from build123d import *

# Parameters (mm, degrees)
F2_DEPTH = 9
F3_COUNT = 8
F4_ANGLE = -12.10395829
F5_R     = 1.5
F6_DEPTH = 9


with BuildPart() as f2:
    # F0 (on Top) → F2 (new body)
    with BuildSketch(Plane.XY):
        with BuildLine():
            ThreePointArc((3.6214284351, 1.6281359465), (-3.8823170623, -0.8325772028), (3.9705881895, 0))
            ThreePointArc((3.9705881895, 0), (3.8823170623, 0.8325772028), (3.6214284351, 1.6281359465))
        make_face()
        with BuildLine():
            ThreePointArc((3.6214284351, 1.6281359465), (3.8823170623, 0.8325772028), (3.9705881895, 0))
            Line((3.9705881895, 0), (4.974843229, 0))
            add(Edge.make_bspline(
                [(4.974843229, 0), (4.9801466314, 0.0001925881), (4.9946353816, 0.0007187334), (5.0515091084, 0.007901301), (5.1389720703, 0.0270949003), (5.2611962602, 0.0647089906), (5.4129160811, 0.1262103484), (5.5914935571, 0.2170132856), (5.7925834332, 0.3418264578), (6.0112959876, 0.5056653333), (6.2248108983, 0.6935311725), (6.3607565303, 0.8389400469), (6.4217785849, 0.9054272978)],
                knots=[0, 0, 0, 0, 0.0334564641, 0.0914021433, 0.1662094232, 0.2547225024, 0.3550868593, 0.4660438076, 0.5866667132, 0.7162364887, 0.8541740412, 0.9672633179, 0.9672633179, 0.9672633179, 0.9672633179], degree=3))
            ThreePointArc((6.4217785849, 0.9054272978), (6.3411178656, 1.3598760973), (6.2283392589, 1.8074370975))
            add(Edge.make_bspline(
                [(4.5373727694, 2.0399297793), (4.5422887796, 2.041928782), (4.5557191847, 2.0473900024), (4.6105368383, 2.0641600629), (4.698178928, 2.0825183873), (4.8250787688, 2.0983298636), (4.9886754487, 2.1044492916), (5.1887830997, 2.0948567755), (5.4233693532, 2.0634759551), (5.6900310606, 2.0037273789), (5.961804421, 1.9199333981), (6.1454202376, 1.843055654), (6.2283392589, 1.8074370975)],
                knots=[0, 0, 0, 0, 0.0334564641, 0.0914021433, 0.1662094232, 0.2547225024, 0.3550868593, 0.4660438076, 0.5866667132, 0.7162364887, 0.8541740412, 0.9672633179, 0.9672633179, 0.9672633179, 0.9672633179], degree=3))
            Line((4.5373727694, 2.0399297793), (3.6214284351, 1.6281359465))
        make_face()
    extrude(amount=F2_DEPTH)

    # F3: F2 ×8 about axis
    f3_axis = Axis((0, 0, 12.9622193053), (0, 0, 1))


with BuildPart() as f2_1:
    add(f2.part)
    for i in range(1, F3_COUNT):
        add(f2.part.rotate(f3_axis, i * 360 / F3_COUNT))


with BuildPart() as f2_2:
    # F4: moved
    add(f2_1.part.rotate(Axis((0, 0, 12.9622193053), (0, 0, 1)), F4_ANGLE))

    # F5 (on face) → F6 (cut, through all)
    with BuildSketch(Plane.XY.offset(9)):
        Circle(F5_R)
    extrude(amount=-F6_DEPTH, mode=Mode.SUBTRACT)


solid = f2_2.part
Could you check a few things on this model? Use its own coordinates, in mm. A direction names the side the tool comes from. Give positions to 0.01 mm unless a question says otherwise; leave off trailing zeros. Order: outer loops, then holes, each group sorted by start corner. A loop starts at its lowest first (then second) coordinate and runs counter-clockwise, first axis right, second up. Notation, with made-up numbers: (21, 38.25) - (52, 38.25) arc R31 ccw to (52, 70.25) - close; hole circle Ø4 at (-13, -34.75). An arc over 180 degrees is marked (long way). One line per question, with ' | ' between items. Start each with the question number.
Item 1: I want a section at C-C on y = -3.5. Give the number of separate pieces and of enclosed holes in the cut face, then the cut area to 3 significant figures.
Item 2: I want a section at A-A on y = 0. Write out the boundary of the cut face in (x, z).
Item 3: I'm going to push flat-ended pins straight in: pin 1 Ø1.5 at (x, z) = (-2.5, 6) entering from -Y; pin 2 Ø1.5 at (y, z) = (-2, 2.5) entering from -X; pin 3 Ø2 at (y, z) = (3, 7) entering from -X. Where does each tip first touch, or does it pass through?
Item 4: Thinking about a two-plate mould opening in Y: for faces 1 (the cylindrical face through (3.672, 1.51, 4.437)), 2 (the cylindrical face through (0.006, 6.485, 4.437)), 3 (the flat face through (-2.43, -3.76, 4.44)), which applies, pulls with the +Y half, pulls with the -Y half, needs draft (parallel to the pull), parting line crosses it, or undercut?
Item 5: For faces 4 (the cylindrical face through (-6.485, 0.006, 4.437)), 5 (the flat face through (-2.425, 3.75, 4.437)), 6 (the flat face through (3.76, -2.43, 4.44)), 7 (the flat face through (4.366, -0.936, 4.437)), 8 (the flat face through (2.425, -3.75, 4.437)), which set-ups out of +Z, -Z, +X, -X, +Y, -Y let a thin tool reach every point of the face, with its end or its side?
Item 6: I need wall thicknesses on probe 1 along Y at (x, z) = (0, 5.5); probe 2 along Y at (x, z) = (4.5, 3.25); probe 3 along X at (y, z) = (-0.5, 7.5). Which ranges of each line are inside material? Lowest first, please. Write a range as [from, to].
Verdict:
1) separate pieces: 3 | enclosed holes: 0 | area: 77.6 mm^2
2) outline: (-6.49, 0) - (-1.5, 0) - (-1.5, 9) - (-6.49, 9) - close; (1.5, 0) - (6.49, 0) - (6.49, 9) - (1.5, 9) - close
3) pin 1: y = -4.59 | pin 2: x = -4.24 | pin 3: x = -4.85
4) face 1: undercut | face 2: pulls with the +Y half | face 3: pulls with the -Y half
5) face 4: +Z, -Z, -X | face 5: +Z, -Z, +Y | face 6: +Z, -Z, +X | face 7: +Z, -Z | face 8: +Z, -Z, -Y
6) probe 1: [-6.49, -1.5], [1.5, 6.49] | probe 2: [-4.67, -3.09], [-0.97, 0.97], [3.09, 4.67] | probe 3: [-6.41, -1.41], [1.41, 6.41]
